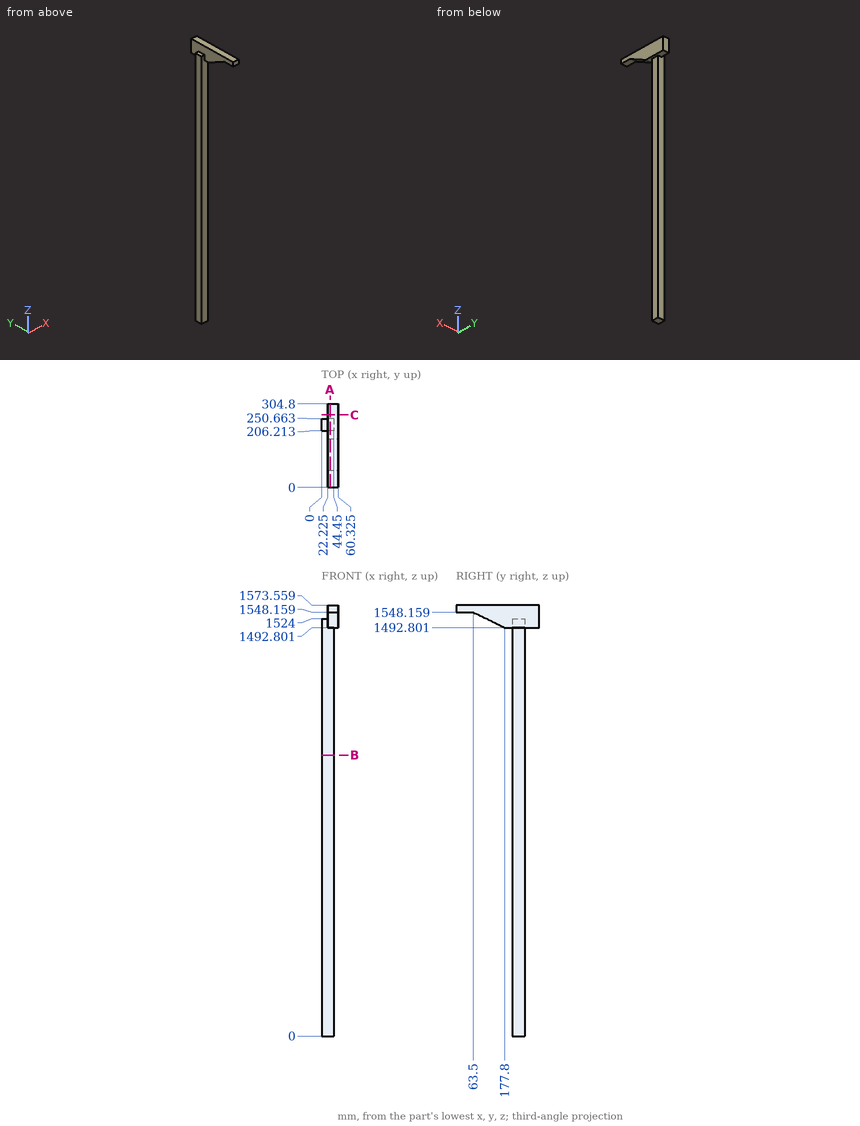
Could you check a few things on this drawing? It's one solid part, dimensions in mm from its lowest x, y, z. Give positions to 0.01 mm unless a question says otherwise; leave off trailing zeros. Order: outer loops, then holes, each group sorted by start corner. A loop starts at its lowest first (then second) coordinate and runs counter-clockwise, first axis right, second up.
1. Suppose I cut it at B-B (z = 1026.5). Write out the boundary of the cut face in (x, y), plus the area to 3 significant figures.
Answers below:
outline: (0, 206.21) - (44.45, 206.21) - (44.45, 250.66) - (0, 250.66) - close
area: 1,980 mm2
2. Suppose I cut it at A-A (x = 31.5). Write out the boundary of the cut face in (y, z).
Answers below:
outline: (0, 1548.16) - (63.5, 1548.16) - (177.8, 1492.8) - (206.21, 1492.8) - (206.21, 0) - (250.66, 0) - (250.66, 1492.8) - (304.8, 1492.8) - (304.8, 1573.56) - (0, 1573.56) - close
3. For pin 1 (2 mm diameter, centred on x = 29.5, z = 591.5, fed in from -Y); pin 2 (2 mm diameter, centred on x = 41, y = 99, fed in from -Z); pin 3 (8 mm diameter, centred on y = 242.5, z = 316.5, fed in from +X), each with a flat end and sliding along its axis, tell me the tip position at first contact or that it passes through.
Answers below:
pin 1: stops at y = 206.21
pin 2: stops at z = 1530.48
pin 3: stops at x = 44.45
4. I need wall thicknesses on L1, parallel to Y at x = 30, z = 1053; L2, parallel to Z at x = 56, y = 285; L3, parallel to Z at x = 32.5, y = 63. Which ranges of each line are inside material? Lowest first, please.
Answers below:
L1: y = 206.21 to 250.66
L2: z = 1492.8 to 1573.56
L3: z = 1548.16 to 1573.56
5. Suppose I cut it at C-C (y = 265). Write out the boundary of the cut face in (x, z) (1 decimal), plus the area to 3 significant figures.
Answers below:
outline: (22.2, 1492.8) - (60.3, 1492.8) - (60.3, 1573.6) - (22.2, 1573.6) - close
area: 3,080 mm2
